Input: part model. Units: mm. Frame: model coordinates. Face numbers are marked on the shaded views. A direction names the side the tool comes from. Coordinates: 2 decimals unless noted, no trailing zeros. Loops run counter-clockwise (first coordinate to the right, second up) from the corner with the lowest first, then second, coordinate; pieces in that order, holes last.
(1) Section A-A, the plane y = 6. Return loops of the section in (x, z).
(2) Section B-B, the plane x = 9. Return loops of the section in (y, z).
(3) Line query: L1, parallel to Y at x = 0, z = 21; L2, parallel to Z at x = -6, y = 0; L3, parallel to Z at x = 3, y = -2.5. Output: solid intervals per line, ascending.
(4) Contact query for flat-ended pins moving along their axis: P1, Ø2.5, axis at x = -15.494, y = 0, coming from the -Z side; P2, Ø2, axis at y = -1, z = -15, coming from the -X side; P3, Ø2, axis at x = 14, z = 20, coming from the +Y side. Output: stop coordinate, or through.
(5) Mould query, pull axis X, two halves, no side actions, for the marked faces 5 and 6. Classes: released by +X, released by -X, zero draft, split by the parting line, or undercut.
(6) Set-up query: the marked faces 1, 2, 3 and 4. Return all of +Z, -Z, +X, -X, +Y, -Y with unobstructed straight access to the full face (end or side cutting, diameter ignored); none if empty.
(7) Section C-C, the plane z = -15. Return loops of the section in (x, y).
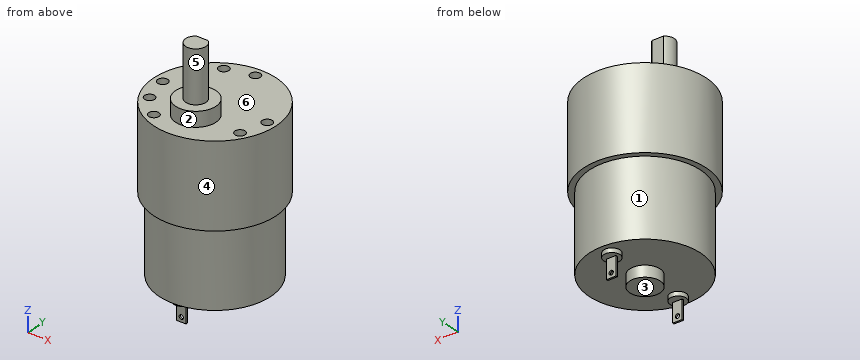
```python
from build123d import *

# Parameters (mm, degrees)
SKETCH1_R           = 18.161
BOSS_EXTRUDE1_DEPTH = 24.511
SKETCH2_R           = 16.51
BOSS_EXTRUDE2_DEPTH = 22.606
SKETCH3_R           = 4.5085
BOSS_EXTRUDE3_DEPTH = 3.302
SKETCH4_R           = 2.413
BOSS_EXTRUDE4_DEPTH = 1.27
SKETCH5_R           = 5.969
BOSS_EXTRUDE5_DEPTH = 4.3688
BOSS_EXTRUDE6_DEPTH = 15.24
SKETCH8_W           = 5.588
SKETCH8_H           = 2.794
SKETCH8_R           = 0.635
BOSS_EXTRUDE7_DEPTH = 0.254
CIRPATTERN1_COUNT   = 2
CIRPATTERN2_COUNT   = 12


with BuildPart() as part:
    # Sketch1 → Boss-Extrude1 (new body)
    with BuildSketch(Plane.XY):
        Circle(SKETCH1_R)
    extrude(amount=BOSS_EXTRUDE1_DEPTH)

    # Sketch2 → Boss-Extrude2 (add)
    with BuildSketch(Plane(origin=(0, 0, 0), x_dir=(-1, 0, 0), z_dir=(0, 0, -1))):
        Circle(SKETCH2_R)
    extrude(amount=BOSS_EXTRUDE2_DEPTH)

    # Sketch3 → Boss-Extrude3 (add)
    with BuildSketch(Plane(origin=(0, 0, -22.606), x_dir=(-1, 0, 0), z_dir=(0, 0, -1))):
        Circle(SKETCH3_R)
    extrude(amount=BOSS_EXTRUDE3_DEPTH)

    # Sketch4 → Boss-Extrude4 (add)
    with BuildSketch(Plane(origin=(0, 0, -22.606), x_dir=(-1, 0, 0), z_dir=(0, 0, -1))):
        with Locations((0, -12.7)):
            Circle(SKETCH4_R)
        with Locations((0, 12.7)):
            Circle(SKETCH4_R)
    extrude(amount=BOSS_EXTRUDE4_DEPTH)

    # Sketch5 → Boss-Extrude5 (add)
    with BuildSketch(Plane.XY.offset(24.511)):
        with Locations((0, -7.366)):
            Circle(SKETCH5_R)
    extrude(amount=BOSS_EXTRUDE5_DEPTH)

    # Sketch6 → Boss-Extrude6 (add)
    with BuildSketch(Plane.XY.offset(28.8798)):
        with BuildLine():
            Line((-1.715657017, -4.905), (1.715657017, -4.905))
            ThreePointArc((1.715657017, -4.905), (0, -10.366), (-1.715657017, -4.905))
        make_face()
    extrude(amount=BOSS_EXTRUDE6_DEPTH)

    # Sketch8 → Boss-Extrude7 (add, symmetric)
    with BuildSketch(Plane.ZX.offset(12.7)):
        with Locations((-26.67, 0)):
            Rectangle(SKETCH8_W, SKETCH8_H)
        with Locations((-28.067, 0)):
            Circle(SKETCH8_R, mode=Mode.SUBTRACT)
    boss_extrude7 = extrude(amount=BOSS_EXTRUDE7_DEPTH, both=True)

    # CirPattern1: Boss-Extrude7 ×2 about axis
    cirpattern1_axis = Axis((0, 0, 0), (0, 0, 1))
    for i in range(1, CIRPATTERN1_COUNT):
        add(boss_extrude7.rotate(cirpattern1_axis, i * 360 / CIRPATTERN1_COUNT))

    # Sketch12 → 3.0mm Dowel Hole1 (revolve, cut)
    with BuildSketch(Plane(origin=(0, 15.494, 24.511), x_dir=(0, -1, 0), z_dir=(1, 0, 0))):
        Polygon((0, 0), (0, 11.061290929), (1.5, 10.16), (1.5, 0), align=None)
    f_3_0mm_dowel_hole1 = revolve(axis=Axis((0, 15.494, 30.861), (0, 0, -1)), mode=Mode.SUBTRACT)

    # CirPattern2: 3.0mm Dowel Hole1 ×12 about axis, 5 skipped
    cirpattern2_axis = Axis((0, 0, 24.511), (0, 0, -1))
    add([f_3_0mm_dowel_hole1.rotate(cirpattern2_axis, i * 360 / CIRPATTERN2_COUNT) for i in range(1, CIRPATTERN2_COUNT) if i not in (1, 2, 5, 6, 10)], mode=Mode.SUBTRACT)


solid = part.part
```
Report:
1. outline: (-17.14, 0) - (-15.38, 0) - (-15.38, -22.61) - (15.38, -22.61) - (15.38, 0) - (17.14, 0) - (17.14, 24.51) - (-17.14, 24.51) - close
2. outline: (-15.77, 0) - (-13.84, 0) - (-13.84, -22.61) - (13.84, -22.61) - (13.84, 0) - (15.77, 0) - (15.77, 24.51) - (-15.77, 24.51) - close
3. L1: y = -18.16 to 13.99, 16.99 to 18.16
3. L2: z = -22.61 to 24.51
3. L3: z = -25.91 to 28.88
4. P1: stops at z = -22.61
4. P2: stops at x = -16.51
4. P3: stops at y = 12.68
5. face 5: split by the parting line
5. face 6: zero draft
6. face 1: -Z
6. face 2: +Z
6. face 3: -Z, +X, -X
6. face 4: +Z, -Z
7. outline: circle Ø33.02 at (0, 0)
